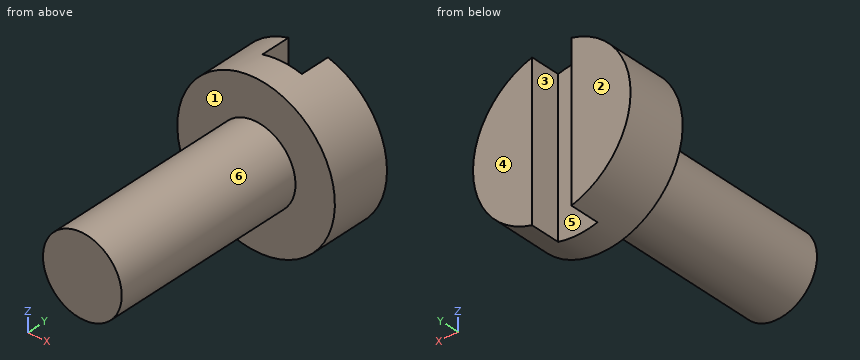
```python
from build123d import *

# Parameters (mm, degrees)
SKETCH1_R          = 4
EXTRUDE1_DEPTH     = 3
CUT_EXTRUDE1_DEPTH = 1.5
SKETCH3_R          = 2
EXTRUDE2_DEPTH     = 10


with BuildPart() as part:
    # Sketch1 → Extrude1 (new body)
    with BuildSketch(Plane(origin=(0, 0, 0), x_dir=(1, 0, 0), z_dir=(0, 1, 0))):
        with Locations(Location((0, 0, 0), (0, 0, 270))):  # turned: the seam where the file's is
            Circle(SKETCH1_R)
    extrude(amount=EXTRUDE1_DEPTH)

    # Sketch2 → Cut-Extrude1 (cut)
    with BuildSketch(Plane(origin=(0, 3, 0), x_dir=(-1, 0, 0), z_dir=(0, 1, 0))):
        Polygon((0, 4.401224563), (-1, 4.401224563), (-1, -5.078336035), (1, -5.078336035), (1, 4.401224563), align=None)
    extrude(amount=-CUT_EXTRUDE1_DEPTH, mode=Mode.SUBTRACT)

    # Sketch3 → Extrude2 (add)
    with BuildSketch(Plane.XZ):
        with Locations(Location((0, 0, 0), (0, 0, 90))):  # turned: the seam where the file's is
            Circle(SKETCH3_R)
    extrude(amount=EXTRUDE2_DEPTH)


solid = part.part
```
Input: part model. Units: mm. Frame: model coordinates. Face numbers are marked on the shaded views. A direction names the side the tool comes from. Give positions to 0.01 mm unless a question says otherwise; leave off trailing zeros. Order: outer loops, then holes, each group sorted by start corner. A loop starts at its lowest first (then second) coordinate and runs counter-clockwise, first axis right, second up. Notation, with made-up numbers: (40.25, 17.5) - (59.25, 17.5) arc R12 ccw to (59.25, 35.5) - close; hole circle Ø3 at (33.5, 32.5). An arc over 180 degrees is marked (long way). Use a Markdown table: item, result.
(1) Pin query (flat end, axial travel): pin 1 (0.8 mm diameter, centred on y = 2.5, z = -1, fed in from -X); pin 2 (0.6 mm diameter, centred on x = 0, z = 0, fed in from +Y); pin 3 (0.8 mm diameter, centred on y = 2, z = 1.5, fed in from +X). Return the tip coordinate at first contact, or that it passes through.
Computed values:
| item | result |
|---|---|
| pin 1 | stops at x = -3.95 |
| pin 2 | stops at y = 1.5 |
| pin 3 | stops at x = 3.85 |
(2) Section query C-C (y = -2). Output: boundary loops of the cut face in (x, z).
Computed values:
| item | result |
|---|---|
| outline | circle Ø4 at (0, 0) |
(3) Draft query along X for the marked faces 4, 5 and 6. Return one class per face: released by +X, released by -X, zero draft, split by the parting line, or undercut.
Computed values:
| item | result |
|---|---|
| face 4 | zero draft |
| face 5 | undercut |
| face 6 | split by the parting line |
(4) Section query B-B (z = 0). Output: boundary loops of the cut face in (x, y).
Computed values:
| item | result |
|---|---|
| outline | (-4, 0) - (-2, 0) - (-2, -10) - (2, -10) - (2, 0) - (4, 0) - (4, 3) - (1, 3) - (1, 1.5) - (-1, 1.5) - (-1, 3) - (-4, 3) - close |
(5) Access query for the marked faces 1, 2 and 3. Directions: +Z, -Z, +X, -X, +Y, -Y. A direction counts if a zero-diameter tool reaches every point of the face in a straight line with its end or side. Return the directions, or none.
Computed values:
| item | result |
|---|---|
| face 1 | -Y |
| face 2 | +Z, -Z, +X, -X, +Y |
| face 3 | +Z, -Z, +Y |
(6) Section query D-D (z = 2.5). Output: boundary loops of the cut face in (x, y), then the cut area to 3 significant figures.
Computed values:
| item | result |
|---|---|
| outline | (-3.12, 0) - (3.12, 0) - (3.12, 3) - (1, 3) - (1, 1.5) - (-1, 1.5) - (-1, 3) - (-3.12, 3) - close |
| area | 15.7 mm2 |
(7) Line query: line 1 (Y direction, x = 2, z = 1.5); line 2 (Y direction, x = -0.75, z = -0.75); line 3 (X direction, y = -8, z = -1). Output: solid intervals per line, ascending. Write a range as from..to.
Computed values:
| item | result |
|---|---|
| line 1 | y = 0..3 |
| line 2 | y = -10..1.5 |
| line 3 | x = -1.73..1.73 |
(8) Section query A-A (x = 0). Output: boundary loops of the cut face in (y, z).
Computed values:
| item | result |
|---|---|
| outline | (-10, -2) - (0, -2) - (0, -4) - (1.5, -4) - (1.5, 4) - (0, 4) - (0, 2) - (-10, 2) - close |
